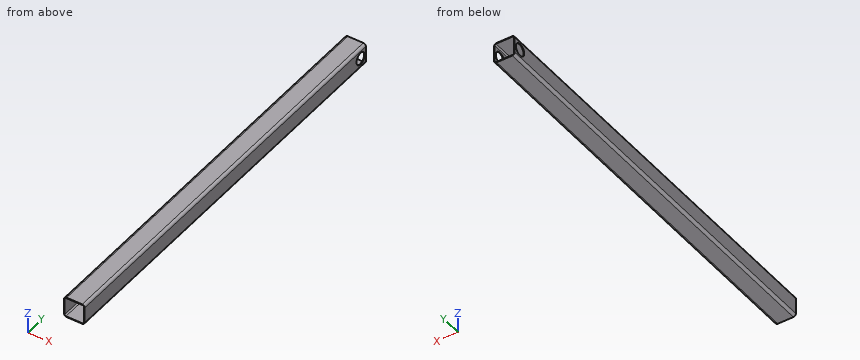
from build123d import *

# Parameters (mm, degrees)
BOSS_EXTRUDE1_DEPTH = 762
SKETCH2_R           = 22.479
CUT_EXTRUDE1_DEPTH  = 77.2


with BuildPart() as part:
    # Sketch1 → Boss-Extrude1 (new body, symmetric)
    with BuildSketch(Plane(origin=(0, 0, 0), x_dir=(1, 0, 0), z_dir=(0, 1, 0))):
        with BuildLine():
            Line((-28.575, -38.1), (28.575, -38.1))
            ThreePointArc((28.575, -38.1), (35.310192091, -35.310192091), (38.1, -28.575))
            Line((38.1, -28.575), (38.1, 28.575))
            ThreePointArc((38.1, 28.575), (35.310192091, 35.310192091), (28.575, 38.1))
            Line((28.575, 38.1), (-28.575, 38.1))
            ThreePointArc((-28.575, 38.1), (-35.310192091, 35.310192091), (-38.1, 28.575))
            Line((-38.1, 28.575), (-38.1, -28.575))
            ThreePointArc((-38.1, -28.575), (-35.310192091, -35.310192091), (-28.575, -38.1))
        make_face()
        with BuildLine():
            Line((-30.9245, -35.687), (30.9245, -35.687))
            ThreePointArc((30.9245, -35.687), (34.292096045, -34.292096045), (35.687, -30.9245))
            Line((35.687, -30.9245), (35.687, 30.9245))
            ThreePointArc((35.687, 30.9245), (34.292096045, 34.292096045), (30.9245, 35.687))
            Line((30.9245, 35.687), (-30.9245, 35.687))
            ThreePointArc((-30.9245, 35.687), (-34.292096045, 34.292096045), (-35.687, 30.9245))
            Line((-35.687, 30.9245), (-35.687, -30.9245))
            ThreePointArc((-35.687, -30.9245), (-34.292096045, -34.292096045), (-30.9245, -35.687))
        make_face(mode=Mode.SUBTRACT)
    extrude(amount=BOSS_EXTRUDE1_DEPTH, both=True)

    # Sketch2 → Cut-Extrude1 (cut, through all)
    with BuildSketch(Plane(origin=(38.1, 0, 0), x_dir=(0, 0, -1), z_dir=(1, 0, 0))):
        with Locations((0, 733.171)):
            Circle(SKETCH2_R)
    extrude(amount=-CUT_EXTRUDE1_DEPTH, mode=Mode.SUBTRACT)


solid = part.part
Could you check a few things on this model? Use its own coordinates, in mm. Give positions to 0.01 mm unless a question says otherwise; leave off trailing zeros. Order: outer loops, then holes, each group sorted by start corner. A loop starts at its lowest first (then second) coordinate and runs counter-clockwise, first axis right, second up. Notation, with made-up numbers: (41.25, 66.25) -> (89.25, 66.25) arc R21 ccw to (89.25, 102.25) -> close; hole circle Ø10 at (43.5, 66.25). An arc over 180 degrees is marked (long way). Return JSON: item names as keys, results as strings.
1. I need wall thicknesses on line 1 (Z direction, x = 24, y = 327); line 2 (Y direction, x = -36.8, z = 0). Which ranges of each line are inside material? Lowest first, please. Write a range as from..to.
Answer list:
{"line 1": "z = -38.1..-35.69, 35.69..38.1", "line 2": "y = -762..710.69, 755.65..762"}
2. Imagine slicing it at C-C on x = -8.5. List the corners of the cut face in (y, z) for me.
Answer list:
{"outline": "(-762, -38.1) -> (762, -38.1) -> (762, -35.69) -> (-762, -35.69) -> close; (-762, 35.69) -> (762, 35.69) -> (762, 38.1) -> (-762, 38.1) -> close"}
3. Imagine slicing it at A-A on z = 0. List the corners of the cut face in (x, y) for me, then the cut area to 3 significant figures.
Answer list:
{"outline": "(-38.1, -762) -> (-35.69, -762) -> (-35.69, 710.69) -> (-38.1, 710.69) -> close; (-38.1, 755.65) -> (-35.69, 755.65) -> (-35.69, 762) -> (-38.1, 762) -> close; (35.69, -762) -> (38.1, -762) -> (38.1, 710.69) -> (35.69, 710.69) -> close; (35.69, 755.65) -> (38.1, 755.65) -> (38.1, 762) -> (35.69, 762) -> close", "area": "7,140 mm2"}
